The listing builds one solid part. Answer for the finished solid, in the listing's coordinates (mm). Round coordinates to 2 decimals unless told otherwise and drop trailing zeros. Loops run counter-clockwise (first coordinate to the right, second up) from the corner with the lowest first, then second, coordinate; pieces in that order, holes last. Notation, with made-up numbers: (35, 41) -> (87, 41) arc R24 cw to (87, 53) -> close; hole circle Ø11 at (53, 3). An arc over 180 degrees is marked (long way). Write each question's results on one line, items separated by ' | '. Start each with the question number.
(1) The part is cut by section D-D (z = 34). Determine the outline of the cut face in (x, y), plus the area to 3 significant figures.
(2) The part is cut by section C-C (y = -2.5). Determine the outline of the cut face in (x, z), plus the area to 3 significant figures.
(3) Straight lines are drawn through the part: probe 1 along X at (y, z) = (-0.5, -26.5); probe 2 along X at (y, z) = (-3.5, -33); probe 3 along Z at (x, y) = (50, -2.5). For each, find the intervals that lie inside material, in ascending order.
(4) Determine the mould class of faces 1 (the face through (15, 0, -6)), 2 (the face through (-41.24, -3.22, 6.28)), 3 (the face through (15, -3, -57.774)), 4 (the face through (29.415, -3.131, -30.206)) for opening direction Z: released by +Z, released by -Z, zero draft, split by the parting line, or undercut.
(5) The part is cut by section B-B (z = -24.5). Determine the outline of the cut face in (x, y).
(6) The part is cut by section A-A (x = 42.5). Determine the outline of the cut face in (y, z), plus the area to 3 significant figures.
```python
from build123d import *

# Parameters (mm, degrees)
F1_DEPTH = 6.35
F2_R     = 12.7
F3_DEPTH = 6.351
F5_D     = 25.4


with BuildPart() as f1:
    # F0 (on Front) → F1 (new body)
    with BuildSketch(Plane.XZ):
        Polygon((53.999179, 43.826219), (-53.950821, 43.826219), (-53.950821, -57.773781), (85.749179, -57.773781), (85.749179, -6.973781), align=None)
    extrude(amount=F1_DEPTH)

    # F2 (on face) → F3 (cut, through all)
    with BuildSketch(Plane.XZ.offset(6.35)):
        with Locations((-28.550821, 5.726219)):
            Circle(F2_R)
    extrude(amount=-F3_DEPTH, mode=Mode.SUBTRACT)

    # F5 (through all)
    with Locations(Plane.XZ.offset(6.35)):
        with Locations((41.528299, -34.020744)):
            Hole(F5_D / 2)


solid = f1.part
```
Checked values:
1) outline: (-53.95, -6.35) -> (60.14, -6.35) -> (60.14, 0) -> (-53.95, 0) -> close | area: 724 mm2
2) outline: (-53.95, -57.77) -> (85.75, -57.77) -> (85.75, -6.97) -> (54, 43.83) -> (-53.95, 43.83) -> close; hole circle Ø25.4 at (-28.55, 5.73); hole circle Ø25.4 at (41.53, -34.02) | area: 12,400 mm2
3) probe 1: x = -53.95 to 31.29, 51.76 to 85.75 | probe 2: x = -53.95 to 28.87, 54.19 to 85.75 | probe 3: z = -57.77 to -43.48, -24.56 to 43.83
4) face 1: zero draft | face 2: undercut | face 3: released by -Z | face 4: undercut
5) outline: (-53.95, -6.35) -> (33.12, -6.35) -> (33.12, 0) -> (-53.95, 0) -> close; (49.93, -6.35) -> (85.75, -6.35) -> (85.75, 0) -> (49.93, 0) -> close
6) outline: (-6.35, -57.77) -> (0, -57.77) -> (0, -46.68) -> (-6.35, -46.68) -> close; (-6.35, -21.36) -> (0, -21.36) -> (0, 43.83) -> (-6.35, 43.83) -> close | area: 484 mm2
